CAD build for the part. Positions are in the model's coordinates, mm. A direction names the side the tool comes from. Coordinates: 2 decimals unless noted, no trailing zeros. Loops run counter-clockwise (first coordinate to the right, second up) from the corner with the lowest first, then second, coordinate; pieces in that order, holes last. Notation, with made-up numbers: M 62.25,40 L 115.25,40 A32 cw 115.25,67 Z; hole C 56,85 d7. An arc over 180 degrees is marked long. Answer as a JSON object with one key per item and string values. Group by question number.
Autodesk Inventor part; units mm, degrees
ref_plane "YZ Plane" through (0, 0, 0) normal (1, 0, 0) x (0, 1, 0)
ref_plane "XZ Plane" through (0, 0, 0) normal (0, 1, 0) x (-1, 0, 0)
ref_plane "XY Plane" through (0, 0, 0) normal (0, 0, 1) x (1, 0, 0)
sketch "Sketch1" plane through (0, 0, 0) normal (1, 0, 0) x (0, 1, 0)
  line L0 (0, 0) -> (80, 0)
  line L1 (80, 0) -> (80, -400)
  line L2 (80, -400) -> (0, -400)
  line L3 (0, -400) -> (0, 0)
  dimension "d0" = 80
  dimension "d1" = 400
extrude "Extrusion1" add sketch "Sketch1" against normal blind 300
sketch "Sketch2" plane through (0, 0, 0) normal (1, 0, 0) x (0, 0, -1)
  circle A0 centre (130, 36.5604) radius 20
  circle A1 centre (200, 36.5604) radius 20
  circle A2 centre (270, 36.5604) radius 20
  line L0 (0, 80) -> (0, 0)
  line L1 (400, 0) -> (400, 80)
  dimension "d4" = 40
  dimension "d5" = 40
  dimension "d6" = 40
  dimension "d7" = 130
  dimension "d8" = 130
  dimension "d9" = 70
extrude "Extrusion2" add sketch "Sketch2" along normal blind 10 contours A0
extrude "Extrusion3" add sketch "Sketch2" along normal blind 10 contours A1
extrude "Extrusion4" add sketch "Sketch2" along normal blind 10 contours A2
sketch "Sketch3" plane through (0, 80, 0) normal (0, 1, 0) x (1, 0, 0)
  circle A0 centre (-140.3312, 200) radius 50
  line L0 (0, 0) -> (-300, 0)
  dimension "d16" = 100
  dimension "d17" = 200
extrude "Extrusion5" add sketch "Sketch3" along normal blind 150
sketch "Sketch4" plane through (-140.3312, 230, -200) normal (0, 1, 0) x (1, 0, 0)
  circle A0 centre (0, 0) radius 20
  point P0 (140.3312, -200)
  dimension "d20" = 40
extrude "Extrusion6" cut sketch "Sketch4" against normal blind 20
sketch "Sketch5" plane through (0, 0, -400) normal (0, -1, 0) x (1, 0, 0)
  line L0 (-75, 350) -> (-75, 50)
  line L1 (-75, 50) -> (-225, 50)
  line L2 (-225, 50) -> (-225, 350)
  line L3 (-225, 350) -> (-75, 350)
  line L4 (0, 400) -> (0, 0)
  line L5 (0, 0) -> (-300, 0)
  dimension "d23" = 300
  dimension "d24" = 150
  dimension "d25" = 300
  dimension "d26" = 75
  dimension "d27" = 50
sketch "Sketch6" plane through (0, 0, -400) normal (0, -1, 0) x (1, 0, 0)
  point P0 (0, 400)
extrude "Extrusion7" add sketch "Sketch5" along normal blind 100
sketch "Sketch7" plane through (0, -100, -400) normal (0, -1, 0) x (1, 0, 0)
  circle A0 centre (-150, 200) radius 30
  line L0 (-225, 50) -> (-75, 50)
  line L1 (-75, 50) -> (-75, 350)
  point P0 (0, 400)
  dimension "d30" = 60
  dimension "d31" = 150
  dimension "d32" = 75
extrude "Extrusion8" add sketch "Sketch7" along normal blind 20
sketch "Sketch8" plane through (-150, -120, -200) normal (0, -1, 0) x (1, 0, 0)
  point P0 (150, 200)
sketch "Sketch9" plane through (0, 0, 0) normal (0, 0, 1) x (1, 0, 0)
  circle A0 centre (-150, 40) radius 25
  line L0 (-300, 0) -> (-300, 80)
  line L1 (0, 80) -> (-300, 80)
  point P0 (0, 0)
  dimension "d35" = 50
  dimension "d36" = 150
  dimension "d37" = 40
extrude "Extrusion9" cut sketch "Sketch9" against normal blind 50
sketch "Sketch10" plane through (0, 0, -400) normal (0, 0, -1) x (-1, 0, 0)
  circle A0 centre (150, 40) radius 25
  circle A1 centre (150, 40) radius 25
  point P0 (0, 0)
extrude "Extrusion10" cut sketch "Sketch10" against normal blind 50
sketch "Sketch11" plane through (-75, 0, -50) normal (1, 0, 0) x (0, 0, -1)
  line L0 (29.0215, -18.1816) -> (279.0215, -18.1816)
  line L1 (279.0215, -18.1816) -> (279.0215, -78.1816)
  line L2 (279.0215, -78.1816) -> (29.0215, -78.1816)
  line L3 (29.0215, -78.1816) -> (29.0215, -18.1816)
  point P0 (-50, 0)
  dimension "d42" = 250
  dimension "d43" = 60
extrude "Extrusion11" cut sketch "Sketch11" against normal blind 10
fillet "Fillet1" radius 4 4 edges at (-85, -48.1816, -329.0215) (-85, -18.1816, -204.0215) (-85, -78.1816, -204.0215) (-85, -48.1816, -79.0215)
sketch "Sketch12" plane through (-300, 0, 0) normal (-1, 0, 0) x (0, 0, 1)
  line L0 (-20.388, 18.3372) -> (-370.388, 18.3372)
  line L1 (-370.388, 18.3372) -> (-370.388, 58.3372)
  line L2 (-370.388, 58.3372) -> (-20.388, 58.3372)
  line L3 (-20.388, 58.3372) -> (-20.388, 18.3372)
  point P0 (0, 0)
  dimension "d47" = 350
  dimension "d48" = 40
extrude "Extrusion12" cut sketch "Sketch12" against normal blind 10
fillet "Fillet2" radius 2 4 edges at (-290, 18.3372, -195.388) (-290, 38.3372, -370.388) (-290, 38.3372, -20.388) (-290, 58.3372, -195.388)
sketch "Sketch13" plane through (-85, 0, -50) normal (1, 0, 0) x (0, 0, -1)
  circle A0 centre (146.4262, -46.2866) radius 20
  point P0 (-50, 0)
  dimension "d52" = 40
extrude "Extrusion13" cut sketch "Sketch13" against normal blind 100
Item 1: Slice it at A-A, the plane z = -38. Write the cut outline in (x, y), then the cut area to 3 significant figures.
Item 2: Pin check, flat tips, straight feed: pin 1 (6 mm diameter, centred on x = -56.5, z = -324.5, fed in from -Y); pin 2 (3 mm diameter, centred on x = -138.5, y = -38, fed in from +Z); pin 3 (12 mm diameter, centred on x = -213.5, z = -97.5, fed in from -Y). Stop position of each tip, or through.
Item 3: Drill centre lines: L1, parallel to X at y = 224.75, z = -200; L2, parallel to Y at x = -11, z = -114; L3, parallel to Y at x = -93, z = -169.5. Where is each one in solid material? Low to high. Write a range as from..to.
Item 4: Slice it at D-D, the plane y = 194.5. Write the cut outline in (x, z).
Item 5: Tool access for faces 1 (the cylindrical face through (-156.503, -109.86, -170.713)), 2 (the cylindrical face through (-155.42, 15.594, -24.65)), 3 (the cylindrical face through (-130, 25, -375)), 4 (the flat face through (-141, 210, -200)): list every direction of +Z, -Z, +X, -X, +Y, -Y with a clear straight run to the whole face (end or side of a thin tool).
Item 6: Pull direction X, two halves, no side cores. Call faces 5 (the cylindrical face through (-94.144, 153.95, -219.15)), 6 (the flat face through (10, 37, -270)), 7 (the flat face through (-150, 40, -350)): released by +X, released by -X, zero draft, split by the parting line, or undercut.
Item 7: Slice it at B-B, the plane z = -270. Write the cut outline in (x, y).
Computed:
{
 "1": {"outline": "M -300,0 L 0,0 L 0,80 L -300,80 L -300,58.34 L -292,58.34 A2 cw -290,56.34 L -290,20.34 A2 cw -292,18.34 L -300,18.34 Z; hole C -150,40 d50", "area": "21,600 mm2"},
 "2": {"pin 1": "y = 0", "pin 2": "z = -50", "pin 3": "y = -100"},
 "3": {"L1": "-190.33..-160.33, -120.33..-90.33", "L2": "0..80", "L3": "-100..80"},
 "4": {"outline": "C -140.33,-200 d100"},
 "5": {"face 1": "-Y", "face 2": "+Z", "face 3": "-Z", "face 4": "+Y"},
 "6": {"face 5": "split by the parting line", "face 6": "released by +X", "face 7": "undercut"},
 "7": {"outline": "M -300,0 L -225,0 L -225,-100 L -75,-100 L -75,-78.18 L -81,-78.18 A4 cw -85,-74.18 L -85,-22.18 A4 cw -81,-18.18 L -75,-18.18 L -75,0 L 0,0 L 0,16.56 L 10,16.56 L 10,56.56 L 0,56.56 L 0,80 L -300,80 L -300,58.34 L -292,58.34 A2 cw -290,56.34 L -290,20.34 A2 cw -292,18.34 L -300,18.34 Z"}
}
